Check sheet for the drawn part. Datum: minimum x, y, z corner. Units: mm. A direction names the side the tool comes from. Give positions to 0.01 mm unless a question says otherwise; leave off trailing zeros. Order: outer loops, then holes, each group sorted by start corner. A loop starts at its lowest first (then second) coordinate and runs counter-clockwise, first axis right, second up.
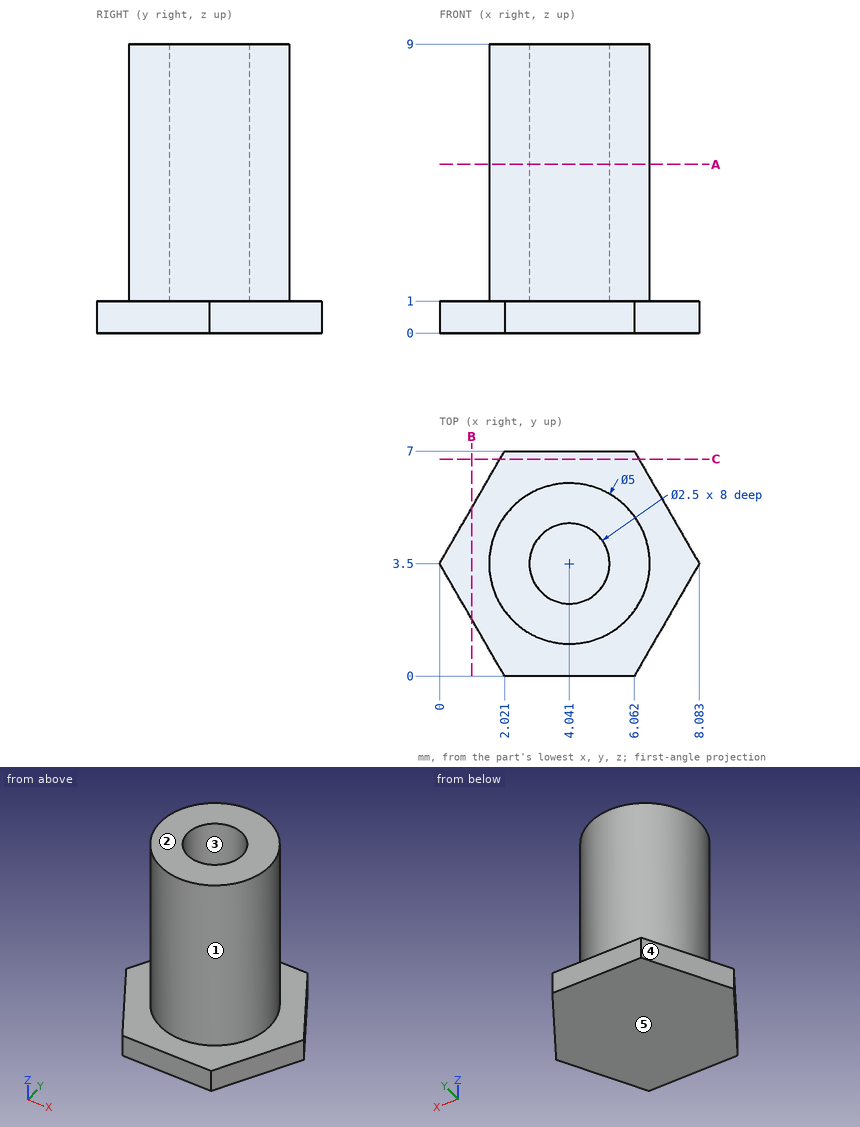
Item 1: Sectioned sample at A-A (z = 5.25). Enter the section's corners in (x, y).
Reported:
outline: circle Ø5 at (4.04, 3.5); hole circle Ø2.5 at (4.04, 3.5)
Item 2: Sectioned sample at B-B (x = 1). Enter the section's corners in (y, z).
Reported:
outline: (1.77, 0) - (5.23, 0) - (5.23, 1) - (1.77, 1) - close
Item 3: Scan lines: L1, parallel to Z at x = 6, y = 5.75; L2, parallel to X at y = 3.75, z = 7.5 (1 decimal); L3, parallel to Y at x = 5, z = 3.5 (1 decimal). Record each from-to range of solid material in increasing order.
Reported:
L1: z = 0 to 1
L2: x = 1.6 to 2.8, 5.3 to 6.5
L3: y = 1.2 to 2.7, 4.3 to 5.8
Item 4: Set-up check for the marked faces 1 and 2: record each of +Z, -Z, +X, -X, +Y, -Y from which the full face is reachable in a straight line by a thin tool's end or side.
Reported:
face 1: +Z
face 2: +Z, +X, -X, +Y, -Y
Item 5: Draft check along X on the marked faces 3, 4 and 5. Enter one of: released by +X, released by -X, zero draft, split by the parting line, or undercut.
Reported:
face 3: undercut
face 4: released by -X
face 5: zero draft
Item 6: Sectioned sample at C-C (y = 6.75). Enter the section's corners in (x, z).
Reported:
outline: (1.88, 0) - (6.21, 0) - (6.21, 1) - (1.88, 1) - close
